```python
from build123d import *

# Parameters (mm, degrees)
F0_R     = 35
F1_DEPTH = 10
F2_R     = 2


with BuildPart() as f1:
    # F0 (on Top) → F1 (new body)
    with BuildSketch(Plane.XY):
        Circle(F0_R)
        with BuildLine():
            ThreePointArc((17.3698096203, 14.3017381376), (19.2313546065, 11.6792551132), (20.7, 8.818163074))
            ThreePointArc((20.7, 8.818163074), (28.1920997883, 6.9713700232), (31.5, 0))
            ThreePointArc((31.5, 0), (28.1920997883, -6.9713700232), (20.7, -8.818163074))
            ThreePointArc((20.7, -8.818163074), (19.045931324, -11.9792528982), (16.9129987609, -14.839153376))
            ThreePointArc((16.9129987609, -14.839153376), (18.2741398317, -17.409907743), (18.7442222222, -20.2805358234))
            ThreePointArc((18.7442222222, -20.2805358234), (10.8508683157, -29.2122397159), (1.016370128, -22.4770325391))
            ThreePointArc((1.016370128, -22.4770325391), (0, -22.5), (-1.016370128, -22.4770325391))
            ThreePointArc((-1.016370128, -22.4770325391), (-13.6419111111, -28.3927501528), (-16.9129987609, -14.839153376))
            ThreePointArc((-16.9129987609, -14.839153376), (-19.045931324, -11.9792528982), (-20.7, -8.818163074))
            ThreePointArc((-20.7, -8.818163074), (-31.5, 0), (-20.7, 8.818163074))
            ThreePointArc((-20.7, 8.818163074), (-19.2313546065, 11.6792551132), (-17.3698096203, 14.3017381376))
            ThreePointArc((-17.3698096203, 14.3017381376), (-14.5251555556, 27.951204913), (-1.7203948242, 22.4341311766))
            ThreePointArc((-1.7203948242, 22.4341311766), (0, 22.5), (1.7203948242, 22.4341311766))
            ThreePointArc((1.7203948242, 22.4341311766), (11.6216169109, 28.8784074582), (19.3751111111, 19.9651463664))
            ThreePointArc((19.3751111111, 19.9651463664), (18.8589865988, 16.9611728797), (17.3698096203, 14.3017381376))
        make_face(mode=Mode.SUBTRACT)
        with BuildLine():
            ThreePointArc((20.7, -8.818163074), (13.5, 0), (20.7, 8.818163074))
            ThreePointArc((20.7, 8.818163074), (19.2313546065, 11.6792551132), (17.3698096203, 14.3017381376))
            ThreePointArc((17.3698096203, 14.3017381376), (6.2250666667, 11.9790878198), (1.7203948242, 22.4341311766))
            ThreePointArc((1.7203948242, 22.4341311766), (0, 22.5), (-1.7203948242, 22.4341311766))
            ThreePointArc((-1.7203948242, 22.4341311766), (-1.4618500193, 21.2116521662), (-1.3751111111, 19.9651463664))
            ThreePointArc((-1.3751111111, 19.9651463664), (-7.3711376244, 11.4812708787), (-17.3698096203, 14.3017381376))
            ThreePointArc((-17.3698096203, 14.3017381376), (-19.2313546065, 11.6792551132), (-20.7, 8.818163074))
            ThreePointArc((-20.7, 8.818163074), (-15.5286299768, 5.6920997883), (-13.5, 0))
            ThreePointArc((-13.5, 0), (-15.5286299768, -5.6920997883), (-20.7, -8.818163074))
            ThreePointArc((-20.7, -8.818163074), (-19.045931324, -11.9792528982), (-16.9129987609, -14.839153376))
            ThreePointArc((-16.9129987609, -14.839153376), (-6.8735941418, -11.750618214), (-0.7442222222, -20.2805358234))
            ThreePointArc((-0.7442222222, -20.2805358234), (-0.8125183297, -21.3871819169), (-1.016370128, -22.4770325391))
            ThreePointArc((-1.016370128, -22.4770325391), (0, -22.5), (1.016370128, -22.4770325391))
            ThreePointArc((1.016370128, -22.4770325391), (5.8465333333, -12.168321494), (16.9129987609, -14.839153376))
            ThreePointArc((16.9129987609, -14.839153376), (19.045931324, -11.9792528982), (20.7, -8.818163074))
        make_face()
    extrude(amount=F1_DEPTH)

    # F2
    f2_edges = [f1.edges().sort_by_distance(p)[0] for p in [
        (-35, 0, 10),
    ]]
    fillet(f2_edges, radius=F2_R)


solid = f1.part
```
Can you work these out from the model? Positions are in its coordinate system, mm. Give positions to 0.01 mm unless a question says otherwise; leave off trailing zeros. Loops run counter-clockwise (first coordinate to the right, second up) from the corner with the lowest first, then second, coordinate; pieces in that order, holes last. Notation, with made-up numbers: M 52,66 L 62,66 A17 cw 62,89 Z; hole C 17,14 d9. An arc over 180 degrees is marked long. Use CSV: the item, a comma, the result in double quotes. Start each with the question number.
1. If I drill on L1, parallel to Y at x = 15, z = 8.25; L2, parallel to X at y = 1, z = 5; L3, parallel to X at y = 14, z = 3, over which ranges is the centre line in solid material (lowest first)?
2. Imagine slicing it at A-A, the plane z = 3.25. Write out the boundary of the cut face in (x, y).
3. Imagine slicing it at B-B, the plane y = 13. Count the separate pieces of the cut face and the enclosed holes in it, plus the area to 3 significant figures.
4. For P1, Ø4, axis at x = 19.5, y = -4.5, coming from the +Z side; P2, Ø1, axis at y = 16, z = 5.5, coming from the +X side; P3, Ø4, axis at y = 17.5, z = 2.5, coming from the -X side; P4, Ø1, axis at y = -8.5, z = 2, coming from the -X side, each with a flat end and sliding along its axis, tell me the tip position at first contact or that it passes through.
Response values:
1,L1,"-31.61 to -27.59, -12.97 to -4.97, 4.97 to 12.24, 27.69 to 31.61"
1,L2,"-34.99 to -31.44, -13.56 to 13.56, 31.44 to 34.99"
1,L3,"-32.08 to -17.11, -3.64 to 3.64, 17.11 to 32.08"
2,outline,"C 0,0 d70; hole C -22.5,0 d18; hole C -10.38,19.97 d18; hole C -9.74,-20.28 d18; hole C 9.74,-20.28 d18; hole C 10.38,19.97 d18; hole C 22.5,0 d18"
3,separate pieces,"3"
3,enclosed holes,"0"
3,area,"420 mm^2"
4,P1,"through"
4,P2,"x = 31.38"
4,P3,"x = -31.38"
4,P4,"x = -34.07"
